For this review, take the finished solid that the model builds, in its own axes (mm). Face numbers are marked on the shaded views. A direction names the side the tool comes from. Round coordinates to 2 decimals unless told otherwise and drop trailing zeros. Write each loop counter-clockwise with the first axis right and the second up, starting at its lowest first coordinate (ties: lowest second). Pieces come first, ordered by that corner, then holes. Notation, with made-up numbers: M 14,-1.75 L 71,-1.75 A9 ccw 71,2.25 Z; hole C 45,42.25 d6. An arc over 180 degrees is marked long. Answer in a Markdown table with one row per item.
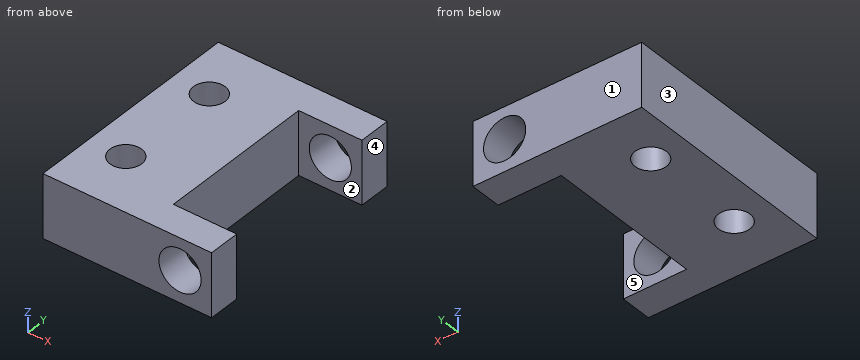
```python
from build123d import *

# Parameters (mm, degrees)
CYLINDER001_R          = 1.5
CYLINDER001_DEPTH      = 10
CYLINDER_R             = 1.5
CYLINDER_DEPTH         = 10
CYLINDER002_R          = 2
CYLINDER002_DEPTH      = 30
CYLINDER002_ROLL_ANGLE = 90
BOX_W                  = 10
BOX_H                  = 15
BOX_DEPTH              = 6
BOX002_W               = 16
BOX002_H               = 3
BOX002_DEPTH           = 6
BOX001_W               = 16
BOX001_H               = 3
BOX001_DEPTH           = 6


with BuildPart() as cylinder001:
    # Cylinder001 → Cylinder001 (new body)
    with BuildSketch(Plane(origin=(3.5, 12.5, 0), x_dir=(1, 0, 0), z_dir=(0, 0, 1))):
        Circle(CYLINDER001_R)
    extrude(amount=CYLINDER001_DEPTH)


with BuildPart() as cylinder:
    # Cylinder → Cylinder (new body)
    with BuildSketch(Plane(origin=(3.5, 2.5, 0), x_dir=(1, 0, 0), z_dir=(0, 0, 1))):
        Circle(CYLINDER_R)
    extrude(amount=CYLINDER_DEPTH)


with BuildPart() as cylinder002:
    # Cylinder002 → Cylinder002 (new body)
    with BuildSketch(Plane.XY):
        Circle(CYLINDER002_R)
    extrude(amount=CYLINDER002_DEPTH)


with BuildPart() as cylinder002_1:
    # Cylinder002 roll: moved
    add(cylinder002.part.rotate(Axis((0, 0, 0), (1, 0, 0)), CYLINDER002_ROLL_ANGLE))


with BuildPart() as cylinder002_2:
    # Cylinder002 placement: moved
    add(cylinder002_1.part.moved(Location((13, 20, 3))))


with BuildPart() as cube:
    # Box → Box (new body)
    with BuildSketch(Plane.XY):
        with Locations((5, 7.5)):
            Rectangle(BOX_W, BOX_H)
    extrude(amount=BOX_DEPTH)


with BuildPart() as cube002:
    # Box002 → Box002 (new body)
    with BuildSketch(Plane(origin=(0, 15, 0), x_dir=(1, 0, 0), z_dir=(0, 0, 1))):
        with Locations((8, 1.5)):
            Rectangle(BOX002_W, BOX002_H)
    extrude(amount=BOX002_DEPTH)


with BuildPart() as cut002:
    # Box001 → Box001 (new body)
    with BuildSketch(Plane(origin=(0, -3, 0), x_dir=(1, 0, 0), z_dir=(0, 0, 1))):
        with Locations((8, 1.5)):
            Rectangle(BOX001_W, BOX001_H)
    extrude(amount=BOX001_DEPTH)

    # Fusion: union Cube, Cube002
    add(cube.part)
    add(cube002.part)

    # Cut: cut Cylinder002
    add(cylinder002_2.part, mode=Mode.SUBTRACT)

    # Cut001: cut Cylinder
    add(cylinder.part, mode=Mode.SUBTRACT)

    # Cut002: cut Cylinder001
    add(cylinder001.part, mode=Mode.SUBTRACT)


solid = cut002.part
```
Q1. Take a section at D-D (y = 2.5). State the section outline as (x, z) points, then the cut area to 3 significant figures.
Found:
| item | result |
|---|---|
| outline | M 0,0 L 2,0 L 2,6 L 0,6 Z; M 5,0 L 10,0 L 10,6 L 5,6 Z |
| area | 42.0 mm² |
Q2. Take a section at A-A (z = 3). State the section outline as (x, y) points, then the cut area to 3 significant figures.
Found:
| item | result |
|---|---|
| outline | M 0,-3 L 11,-3 L 11,0 L 10,0 L 10,15 L 11,15 L 11,18 L 0,18 Z; M 15,-3 L 16,-3 L 16,0 L 15,0 Z; M 15,15 L 16,15 L 16,18 L 15,18 Z; hole C 3.5,2.5 d3; hole C 3.5,12.5 d3 |
| area | 208 mm² |
Q3. Mouldability with a two-part tool opening along Y and no side actions: class the marked faces 1, 2 and 3 as +Y half, -Y half, draft (parallel to the pull), parting line (faces both ways), or undercut.
Found:
| item | result |
|---|---|
| face 1 | +Y half |
| face 2 | undercut |
| face 3 | draft |
Q4. Machinability: for the marked faces 4 and 5, which of the approach directions +Z, -Z, +X, -X, +Y, -Y give a long, thin tool a straight path to every point of the face, cutting with its end or side? Answer none if there is none.
Found:
| item | result |
|---|---|
| face 4 | +Z, -Z, +X, +Y, -Y |
| face 5 | +Z, -Z, +X |
Q5. Insertion check: P1, Ø1.8, axis at x = 3.5, y = 2.5, coming from the -Z side. The pin has a flat end and moves straight along its axis. Give the tip position at first contact, or say it passes through.
Found:
| item | result |
|---|---|
| P1 | through |
Q6. Take a section at C-C (x = 3.5). State the section outline as (y, z) points.
Found:
| item | result |
|---|---|
| outline | M -3,0 L 1,0 L 1,6 L -3,6 Z; M 4,0 L 11,0 L 11,6 L 4,6 Z; M 14,0 L 18,0 L 18,6 L 14,6 Z |
Q7. Take a section at B-B (x = 13). State the section outline as (y, z) points.
Found:
| item | result |
|---|---|
| outline | M -3,0 L 0,0 L 0,1 L -3,1 Z; M -3,5 L 0,5 L 0,6 L -3,6 Z; M 15,0 L 18,0 L 18,1 L 15,1 Z; M 15,5 L 18,5 L 18,6 L 15,6 Z |
Q8. For probe 1 along Y at (x, z) = (3.5, 3.95); probe 2 along Z at (x, y) = (13, 17.1); probe 3 along X at (y, z) = (12.5, 3.1), list the stretches that pass through material, from the lowest coordinate up.
Found:
| item | result |
|---|---|
| probe 1 | -3 to 1, 4 to 11, 14 to 18 |
| probe 2 | 0 to 1, 5 to 6 |
| probe 3 | 0 to 2, 5 to 10 |
